Design review of the part built by this model. Coordinates are the model's own, in mm. Coordinates: 2 decimals unless noted, no trailing zeros. Write each loop counter-clockwise with the first axis right and the second up, starting at its lowest first coordinate (ties: lowest second). Pieces come first, ordered by that corner, then holes. Notation, with made-up numbers: (53.5, 30.5) - (87.5, 30.5) arc R22 cw to (87.5, 42.5) - close; hole circle Ø11 at (-33.75, 59). An arc over 180 degrees is marked (long way). Answer as a JSON object with one key per item and string values.
```python
from build123d import *

# Parameters (mm, degrees)
SKETCH_1_R          = 1
EXTRUDE_1_DEPTH     = 0.8
SKETCH_2_R          = 0.25
CUT_EXTRUDE_1_DEPTH = 3


with BuildPart() as part:
    # Эскиз1 → Вытянуть1 (new body)
    with BuildSketch(Plane.XY):
        Polygon((2, 12.549502762), (3, 12.549502762), (3, 14.849502762), (4, 14.849502762), (4, 16.849502762), (3.25, 16.849502762), (3.25, 24.249502762), (1.75, 25.749502762), (-1.75, 25.749502762), (-3.25, 24.249502762), (-3.25, 16.849502762), (-4, 16.849502762), (-4, 14.849502762), (-3, 14.849502762), (-3, 12.549502762), (-2, 12.549502762), (-2, 16.949502762), (2, 16.949502762), align=None)
        with Locations((0, 22.349502762)):
            Circle(SKETCH_1_R, mode=Mode.SUBTRACT)
    extrude(amount=EXTRUDE_1_DEPTH)

    # Эскиз2 → Вырез-Вытянуть1 (cut)
    with BuildSketch(Plane.XZ.offset(-12.549502762)):
        with Locations(Location((2.5, 0.4, 0), (0, 0, 270))):
            Circle(SKETCH_2_R)
        with Locations(Location((-2.5, 0.4, 0), (0, 0, 90))):
            Circle(SKETCH_2_R)
    extrude(amount=-CUT_EXTRUDE_1_DEPTH, mode=Mode.SUBTRACT)


solid = part.part
```
(1) The part is to be moulded in two halves that separate along X. For faces 1 (the face through (2.5, 25, 0.4)), 2 (the face through (-0.13, 23.34, 0.39)), 3 (the face through (0, 21, 0)), 4 (the face through (-2.5, 25, 0.4)), say which applies: pulls with the +X half, pulls with the -X half, needs draft (parallel to the pull), parting line crosses it, or undercut.
Solved:
{"face 1": "pulls with the +X half", "face 2": "undercut", "face 3": "needs draft", "face 4": "pulls with the -X half"}
(2) Take a section at A-A, the plane y = 15.25. Write out the cut boundary in (x, z), and give its area (3 significant figures).
Solved:
{"outline": "(-4, 0) - (-2, 0) - (-2, 0.8) - (-4, 0.8) - close; (2, 0) - (4, 0) - (4, 0.8) - (2, 0.8) - close; hole circle Ø0.5 at (-2.5, 0.4); hole circle Ø0.5 at (2.5, 0.4)", "area": "2.81 mm^2"}
(3) Take a section at B-B, the plane x = 0. Write out the cut boundary in (y, z), and give its area (3 significant figures).
Solved:
{"outline": "(16.95, 0) - (21.35, 0) - (21.35, 0.8) - (16.95, 0.8) - close; (23.35, 0) - (25.75, 0) - (25.75, 0.8) - (23.35, 0.8) - close", "area": "5.44 mm^2"}
(4) To check wall thickness, follow line 1 (X direction, y = 13.25, z = 0.7); line 2 (X direction, y = 14.95, z = 0.4); line 3 (X direction, y = 14.6, z = 0.4). State the ranges of each line that lie inside material, in increasing order. Write a range as from..to.
Solved:
{"line 1": "x = -3..-2, 2..3", "line 2": "x = -4..-2.75, -2.25..-2, 2..2.25, 2.75..4", "line 3": "x = -3..-2.75, -2.25..-2, 2..2.25, 2.75..3"}
(5) Take a section at D-D, the plane y = 23.75. Write out the cut boundary in (x, z), and give its area (3 significant figures).
Solved:
{"outline": "(-3.25, 0) - (3.25, 0) - (3.25, 0.8) - (-3.25, 0.8) - close", "area": "5.20 mm^2"}
(6) Take a section at C-C, the plane z = 0.4. Write out the cut boundary in (x, y), and give its area (3 significant figures).
Solved:
{"outline": "(-4, 14.85) - (-3, 14.85) - (-3, 12.55) - (-2.75, 12.55) - (-2.75, 15.55) - (-2.25, 15.55) - (-2.25, 12.55) - (-2, 12.55) - (-2, 16.95) - (2, 16.95) - (2, 12.55) - (2.25, 12.55) - (2.25, 15.55) - (2.75, 15.55) - (2.75, 12.55) - (3, 12.55) - (3, 14.85) - (4, 14.85) - (4, 16.85) - (3.25, 16.85) - (3.25, 24.25) - (1.75, 25.75) - (-1.75, 25.75) - (-3.25, 24.25) - (-3.25, 16.85) - (-4, 16.85) - close; hole circle Ø2 at (0, 22.35)", "area": "61.7 mm^2"}
